The model under review builds one solid part; all positions refer to its coordinate system, in mm. Round coordinates to 2 decimals unless told otherwise and drop trailing zeros. Order: outer loops, then holes, each group sorted by start corner. A loop starts at its lowest first (then second) coordinate and runs counter-clockwise, first axis right, second up.
1) Consider section A-A (y = 0). Give the boundary of the cut face in (x, z), then the cut area to 3 significant figures.
2) Consider section B-B (z = -8). Give the boundary of the cut face in (x, y).
3) Consider section C-C (z = 0). Give the boundary of the cut face in (x, y), then the cut area to 3 significant figures.
4) To check wall thickness, follow L1, parallel to Y at x = 0.3, z = -9.5; L2, parallel to Y at x = 2.1, z = -1; L3, parallel to Z at x = -2.05, y = 10. State the ranges of each line that lie inside material, in increasing order.
5) Mouldability with a two-part tool opening along Y and no side actions: class faces 1 (the face through (0, -22, -18.2)), 2 (the face through (-2.5, 10, 17)), 3 (the face through (-0.035, 33.966, 0.521)) as pulls with the +Y half, pulls with the -Y half, needs draft (parallel to the pull), parting line crosses it, or undercut.
6) Clearance check with a flat-ended pin moving along its axis: P1, Ø2, axis at x = 0.5, z = 5, coming from the +Y side. State where the tip first meets the part, or that it passes through.
from build123d import *

# Parameters (mm, degrees)
SKETCH1_R           = 19.5
SKETCH1_R_2         = 4
BOSS_EXTRUDE1_DEPTH = 2.5


with BuildPart() as part:
    # Sketch1 → Boss-Extrude1 (new, symmetric)
    with BuildSketch(Plane.YZ):
        with BuildLine():
            Line((-35.133333333, 13.024933354), (-9.166666667, 23.258809562))
            ThreePointArc((-9.166666667, 23.258809562), (0, 25), (9.166666667, 23.258809562))
            Line((9.166666667, 23.258809562), (35.133333333, 13.024933354))
            ThreePointArc((35.133333333, 13.024933354), (44, 0), (35.133333333, -13.024933354))
            Line((35.133333333, -13.024933354), (9.166666667, -23.258809562))
            ThreePointArc((9.166666667, -23.258809562), (0, -25), (-9.166666667, -23.258809562))
            Line((-9.166666667, -23.258809562), (-35.133333333, -13.024933354))
            ThreePointArc((-35.133333333, -13.024933354), (-44, 0), (-35.133333333, 13.024933354))
        make_face()
        with Locations(Location((0, 0, 0), (0, 0, 270))):
            Circle(SKETCH1_R, mode=Mode.SUBTRACT)
        with Locations(Location((30, 0, 0), (0, 0, 270))):
            Circle(SKETCH1_R_2, mode=Mode.SUBTRACT)
        with Locations(Location((-30, 0, 0), (0, 0, 270))):
            Circle(SKETCH1_R_2, mode=Mode.SUBTRACT)
    extrude(amount=BOSS_EXTRUDE1_DEPTH, both=True)


solid = part.part
Answer below:
1. outline: (-2.5, -25) - (2.5, -25) - (2.5, -19.5) - (-2.5, -19.5) - close; (-2.5, 19.5) - (2.5, 19.5) - (2.5, 25) - (-2.5, 25) - close
1. area: 55.0 mm2
2. outline: (-2.5, -41.49) - (2.5, -41.49) - (2.5, -17.78) - (-2.5, -17.78) - close; (-2.5, 17.78) - (2.5, 17.78) - (2.5, 41.49) - (-2.5, 41.49) - close
3. outline: (-2.5, -44) - (2.5, -44) - (2.5, -34) - (-2.5, -34) - close; (-2.5, -26) - (2.5, -26) - (2.5, -19.5) - (-2.5, -19.5) - close; (-2.5, 19.5) - (2.5, 19.5) - (2.5, 26) - (-2.5, 26) - close; (-2.5, 34) - (2.5, 34) - (2.5, 44) - (-2.5, 44) - close
3. area: 165 mm2
4. L1: y = -40.28 to -17.03, 17.03 to 40.28
4. L2: y = -43.96 to -33.87, -26.13 to -19.47, 19.47 to 26.13, 33.87 to 43.96
4. L3: z = -22.93 to -16.74, 16.74 to 22.93
5. face 1: pulls with the -Y half
5. face 2: needs draft
5. face 3: undercut
6. P1: stops at y = 43.42
